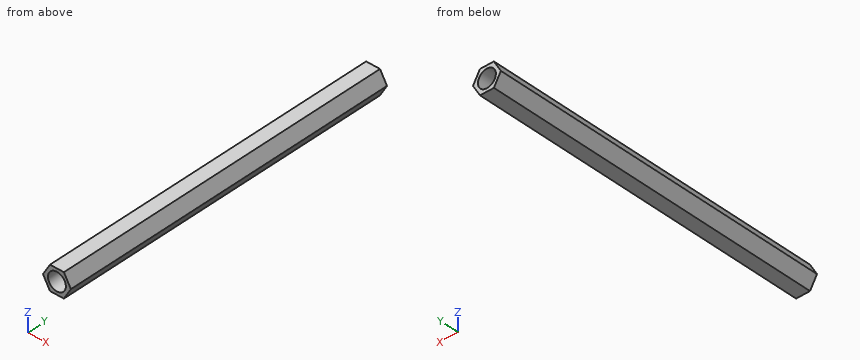
```python
from build123d import *

# Parameters (mm, degrees)
EXTRUDE_1_DEPTH     = 100
SKETCH_2_R          = 2.6
CUT_EXTRUDE_1_DEPTH = 101
SKETCH_3_R          = 2.6
EXTRUDE_2_DEPTH     = 80


with BuildPart() as part:
    # 草图1 → 凸台-拉伸1 (new body)
    with BuildSketch(Plane(origin=(0, 0, 0), x_dir=(1, 0, 0), z_dir=(0, 1, 0))):
        Polygon((4.041451884, 0), (2.020725942, 3.5), (-2.020725942, 3.5), (-4.041451884, 0), (-2.020725942, -3.5), (2.020725942, -3.5), align=None)
    extrude(amount=EXTRUDE_1_DEPTH)

    # 草图2 → 切除-拉伸1 (cut, through all)
    with BuildSketch(Plane(origin=(0, 100, 0), x_dir=(1, 0, 0), z_dir=(0, 1, 0))):
        Circle(SKETCH_2_R)
    extrude(amount=-CUT_EXTRUDE_1_DEPTH, mode=Mode.SUBTRACT)

    # 草图3 → 凸台-拉伸2 (add)
    with BuildSketch(Plane(origin=(0, 90, 0), x_dir=(1, 0, 0), z_dir=(0, 1, 0))):
        Circle(SKETCH_3_R)
    extrude(amount=-EXTRUDE_2_DEPTH)


solid = part.part
```
Input: part model. Units: mm. Frame: model coordinates. Coordinates: 2 decimals unless noted, no trailing zeros. Write each loop counter-clockwise with the first axis right and the second up, starting at its lowest first coordinate (ties: lowest second). Pieces come first, ordered by that corner, then holes. Notation, with made-up numbers: (53, -14.5) -> (87, -14.5) arc R34 ccw to (87, 21.5) -> close; hole circle Ø5 at (22.25, 6.25). An arc over 180 degrees is marked (long way). Write each question's results on one line, items separated by ' | '.
Item 1: Pin query (flat end, axial travel): pin 1 Ø2.5 at (x, z) = (0.5, 0) entering from -Y. Return the tip coordinate at first contact, or that it passes through.
Conclusion:
pin 1: stops at y = 10
Item 2: Section query B-B on x = 0. Return loops of the section in (y, z), plus the area to 3 significant figures.
Conclusion:
outline: (0, -3.5) -> (100, -3.5) -> (100, -2.6) -> (90, -2.6) -> (90, 2.6) -> (100, 2.6) -> (100, 3.5) -> (0, 3.5) -> (0, 2.6) -> (10, 2.6) -> (10, -2.6) -> (0, -2.6) -> close | area: 596 mm^2
Item 3: Section query A-A on y = 62. Return loops of the section in (x, z), plus the area to 3 significant figures.
Conclusion:
outline: (-4.04, 0) -> (-2.02, -3.5) -> (2.02, -3.5) -> (4.04, 0) -> (2.02, 3.5) -> (-2.02, 3.5) -> close | area: 42.4 mm^2
Item 4: Material intervals for probe 1 along Z at (x, y) = (0, 3.75); probe 2 along X at (y, z) = (5.75, 0); probe 3 along Y at (x, z) = (-1, 1.25), sorted ascending.
Conclusion:
probe 1: z = -3.5 to -2.6, 2.6 to 3.5 | probe 2: x = -4.04 to -2.6, 2.6 to 4.04 | probe 3: y = 10 to 90
